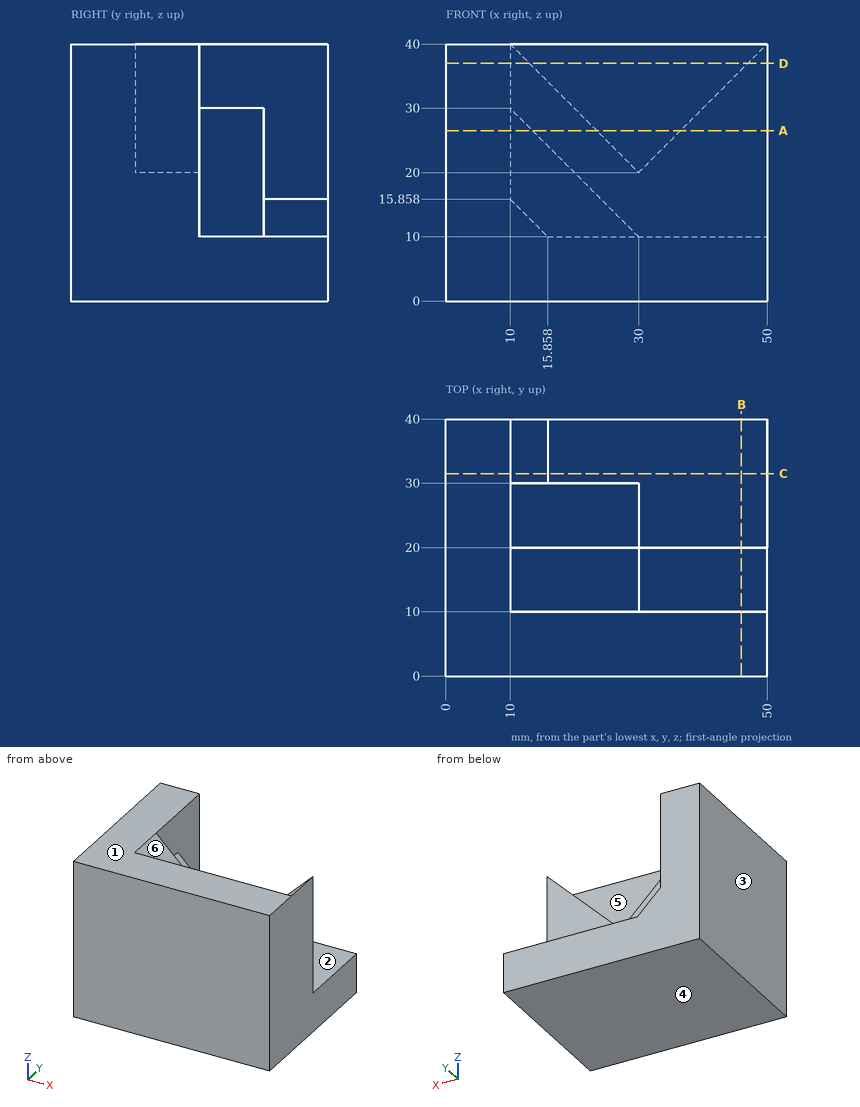
Print and shaded views of the part. All mm, measured from the part's lowest x, y and z. A direction names the side the tool comes from. Round coordinates to 2 decimals unless told otherwise and drop trailing zeros. Loops run counter-clockwise (first coordinate to the right, second up) from the corner with the lowest first, then second, coordinate; pieces in that order, holes last. Notation, with made-up numbers: M 31,4 L 51,4 A26 ccw 51,31 Z; hole C 37.5,56 d8. An arc over 180 degrees is marked long. One line per question, with ' | ' between items.
1) Band-saw the part on C-C (y = 31.5). Give the cut face in (x, z), then the cut area to 3 significant figures.
Solved:
outline: M 0,0 L 50,0 L 50,10 L 15.86,10 L 10,15.86 L 10,40 L 0,40 Z | area: 817 mm²
2) Band-saw the part on D-D (z = 37). Give the cut face in (x, y), then the cut area to 3 significant figures.
Solved:
outline: M 0,0 L 50,0 L 50,20 L 47,20 L 47,10 L 13,10 L 13,20 L 10,20 L 10,40 L 0,40 Z | area: 860 mm²
3) Flat gauge pins, fed straight in: pin 1 (8 mm diameter, centred on x = 44, y = 23, fed in from +Z) (1 decimal); pin 2 (16 mm diameter, centred on x = 25.5, z = 27.5, fed in from +Y); pin 3 (16 mm diameter, centred on x = 22.5, z = 18.5, fed in from +Y). Where does each tip first touch, or does it go through?
Solved:
pin 1: stops at z = 36.6 | pin 2: stops at y = 20 | pin 3: stops at y = 30
4) Band-saw the part on A-A (z = 26.5). Give the cut face in (x, y), then the cut area to 4 significant figures.
Solved:
outline: M 0,0 L 50,0 L 50,20 L 36.5,20 L 36.5,10 L 23.5,10 L 23.5,20 L 13.5,20 L 13.5,30 L 10,30 L 10,40 L 0,40 Z | area: 1,105 mm²
5) Band-saw the part on B-B (x = 46). Give the cut face in (y, z), then the cut area to 3 significant figures.
Solved:
outline: M 0,0 L 40,0 L 40,10 L 20,10 L 20,36 L 10,36 L 10,40 L 0,40 Z | area: 960 mm²
6) 3-axis set-ups, long thin cutter, end or side, ignore diameter. For the marked faces 1 and 2: which of +Z, -Z, +X, -X, +Y, -Y reach the whole face in a straight line?
Solved:
face 1: +Z, +X, -X, +Y, -Y | face 2: +Z, +X, +Y
7) Mould opens along X. For the marked faces 3, 4, 5 and 6 say: +X half, -X half, draft (parallel to the pull), parting line (faces both ways), or undercut.
Solved:
face 3: -X half | face 4: draft | face 5: undercut | face 6: undercut
8) Drill centre lines: line 1 along Y through (x, z) = (27.5, 14); line 2 along Z through (x, y) = (27, 38). Where is each one in solid material? Low to high.
Solved:
line 1: y = 0 to 20 | line 2: z = 0 to 10
